Input: part model. Units: mm. Frame: model coordinates. Face numbers are marked on the shaded views. A direction names the side the tool comes from. Coordinates: 2 decimals unless noted, no trailing zeros. Loops run counter-clockwise (first coordinate to the right, second up) from the corner with the lowest first, then second, coordinate; pieces in that order, holes last. Notation, with made-up numbers: (47.25, -25) -> (52.25, -25) arc R13 cw to (52.25, -15) -> close; hole circle Ø5 at (-23.75, -11.5). An arc over 180 degrees is marked (long way). Put each result on its own line as item: value. Start each with the question number.
1) Cut plane A-A (x = 0.25). Return the cut outline in (y, z), plus the area to 3 significant figures.
2) Pull-direction query (X, two-part tool) for the marked faces 1, 2 and 3; classes: pulls with the +X half, pulls with the -X half, needs draft (parallel to the pull), parting line crosses it, or undercut.
3) Cut plane B-B (z = 0). Return the cut outline in (x, y).
4) Set-up query: the marked faces 4 and 5. Return all of +Z, -Z, +X, -X, +Y, -Y with unobstructed straight access to the full face (end or side cutting, diameter ignored); none if empty.
5) Cut plane D-D (z = 3). Return the cut outline in (x, y), plus the area to 3 significant figures.
6) Material intervals for L1, parallel to X at y = -2, z = 0; L2, parallel to X at y = -5.25, z = -2; L3, parallel to Y at x = -1.75, z = 2, sorted ascending.
7) Cut plane C-C (x = 1.5). Return the cut outline in (y, z), plus the area to 3 significant figures.
8) Contact query for a flat-ended pin moving along its axis: P1, Ø5, axis at y = -10, z = 0, coming from the +X side. Output: stop coordinate, or through.
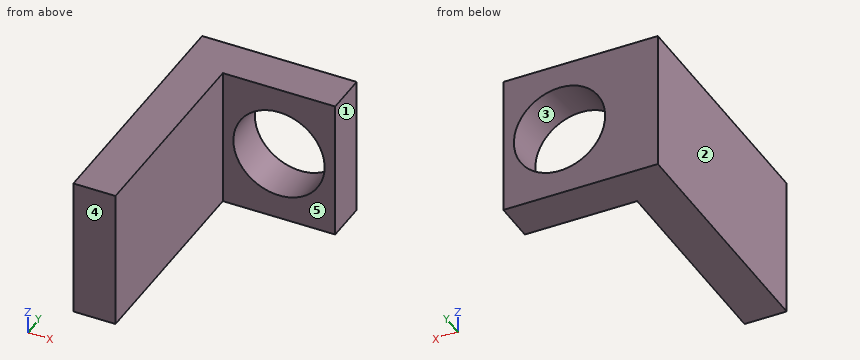
from build123d import *

# Parameters (mm, degrees)
SKETCH1_W           = 8
SKETCH1_H           = 10
SKETCH1_R           = 1.5
BOSS_EXTRUDE1_DEPTH = 3
SKETCH2_W           = 3
SKETCH2_H           = 10
BOSS_EXTRUDE2_DEPTH = 18
SKETCH3_R           = 3.25
CUT_EXTRUDE1_DEPTH  = 3.2


with BuildPart() as part:
    # Sketch1 → Boss-Extrude1 (new body)
    with BuildSketch(Plane(origin=(0, 0, 0), x_dir=(1, 0, 0), z_dir=(0, 1, 0))):
        with Locations((1.5, 0)):
            Rectangle(SKETCH1_W, SKETCH1_H)
        with Locations(Location((1.5, 0, 0), (0, 0, 270))):
            Circle(SKETCH1_R, mode=Mode.SUBTRACT)
    extrude(amount=-BOSS_EXTRUDE1_DEPTH)

    # Sketch2 → Boss-Extrude2 (add)
    with BuildSketch(Plane(origin=(0, 0, 0), x_dir=(1, 0, 0), z_dir=(0, 1, 0))):
        with Locations((-4, 0)):
            Rectangle(SKETCH2_W, SKETCH2_H)
    extrude(amount=-BOSS_EXTRUDE2_DEPTH)

    # Sketch3 → Cut-Extrude1 (cut)
    with BuildSketch(Plane(origin=(0, 0, 0), x_dir=(1, 0, 0), z_dir=(0, 1, 0))):
        with Locations(Location((1.5, 0, 0), (0, 0, 270))):
            Circle(SKETCH3_R)
    extrude(amount=-CUT_EXTRUDE1_DEPTH, mode=Mode.SUBTRACT)


solid = part.part
Results found:
1. outline: (-3, -5) -> (0, -5) -> (0, -3) -> (-3, -3) -> close; (-3, 3) -> (0, 3) -> (0, 5) -> (-3, 5) -> close
1. area: 12.0 mm2
2. face 1: pulls with the +X half
2. face 2: pulls with the -X half
2. face 3: undercut
3. outline: (-5.5, -18) -> (-2.5, -18) -> (-2.5, -3) -> (-1.75, -3) -> (-1.75, 0) -> (-5.5, 0) -> close; (4.75, -3) -> (5.5, -3) -> (5.5, 0) -> (4.75, 0) -> close
4. face 4: +Z, -Z, +X, -X, -Y
4. face 5: +Z, -Z, +X, -Y
5. outline: (-5.5, -18) -> (-2.5, -18) -> (-2.5, -3) -> (0.25, -3) -> (0.25, 0) -> (-5.5, 0) -> close; (2.75, -3) -> (5.5, -3) -> (5.5, 0) -> (2.75, 0) -> close
5. area: 70.5 mm2
6. L1: x = -5.5 to -1.75, 4.75 to 5.5
6. L2: x = -5.5 to -2.5
6. L3: y = -3 to 0
7. outline: (-3, -5) -> (0, -5) -> (0, -3.25) -> (-3, -3.25) -> close; (-3, 3.25) -> (0, 3.25) -> (0, 5) -> (-3, 5) -> close
7. area: 10.5 mm2
8. P1: stops at x = -2.5
